Answer from the drawing. Dimensions are ordinates in mm from the lowest x, y and z of the part. A direction names the side the tool comes from. Coordinates: 2 decimals unless noted, no trailing zeros. Write each loop counter-clockwise with the first axis right and the second up, starting at its lowest first coordinate (ties: lowest second). Pieces come first, ordered by that corner, then holes. Notation, with made-up numbers: M -7.75,87.5 L 15.25,87.5 A28 cw 15.25,106.5 Z; hole C 53.5,-26.5 d4. An arc over 180 degrees is marked long. Put each result on its own line as item: value. Start each with the question number.
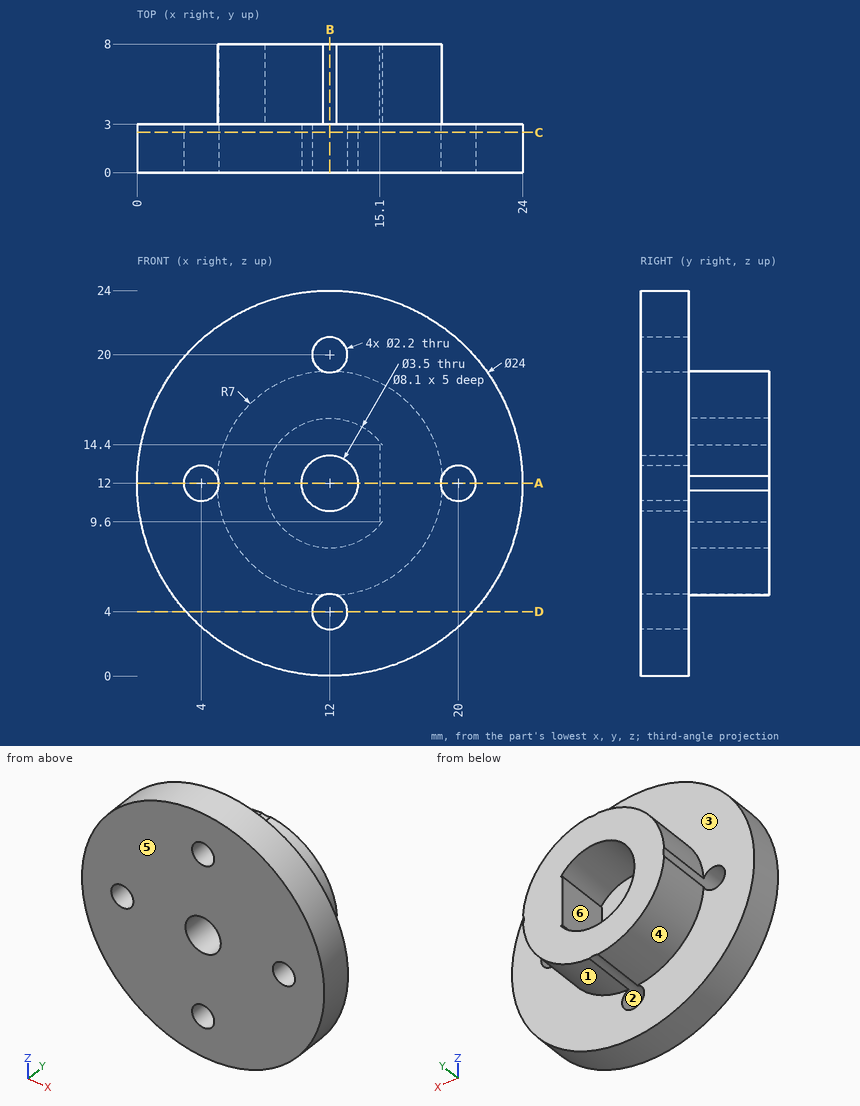
1) Straight lines are drawn through the part: probe 1 along Z at (x, y) = (12, 6); probe 2 along Y at (x, z) = (12.5, 14.5); probe 3 along X at (y, z) = (6.25, 10.25). For each, find the intervals that lie inside material, in ascending order.
2) A cutting plane is placed at A-A on z = 12. Write down the section's boundary in (x, y).
3) A cutting plane is placed at D-D on z = 4. Write down the section's boundary in (x, y).
4) For the marked faces 1, 2 and 3, determine the directions among +Z, -Z, +X, -X, +Y, -Y from which every point of the face is accessible in a straight line to the end or side of a thin tool.
5) Given pin 1 Ø3 at (x, z) = (12, 12) entering from -Y; pin 2 Ø1.5 at (x, y) = (13, 6.5) entering from +Z; pin 3 Ø1 at (y, z) = (1.5, 6) entering from +X; pin 4 Ø2 at (x, z) = (19, 5) entering from +Y, each flat-ended and moving along its own axis, determine where each tip first touches the part or whether it passes through.
6) A cutting plane is placed at C-C on y = 2.5. Write down the section's boundary in (x, z), then the cut area to 3 significant figures.
7) A cutting plane is placed at B-B on x = 12. Write down the section's boundary in (y, z).
8) Determine the mould class of the marked faces 4, 5 and 6 for opening direction X: +X half, -X half, draft (parallel to the pull), parting line (faces both ways), or undercut.
Answers follow:
1. probe 1: z = 5.1 to 7.95, 16.05 to 18.9
1. probe 2: y = 0 to 3
1. probe 3: x = 5.22 to 8.35, 15.1 to 18.78
2. outline: M 0,0 L 2.9,0 L 2.9,3 L 0,3 Z; M 5.1,0 L 10.25,0 L 10.25,3 L 7.95,3 L 7.95,8 L 5.1,8 Z; M 13.75,0 L 18.9,0 L 18.9,8 L 15.1,8 L 15.1,3 L 13.75,3 Z; M 21.1,0 L 24,0 L 24,3 L 21.1,3 Z
3. outline: M 3.06,0 L 10.9,0 L 10.9,3 L 3.06,3 Z; M 13.1,0 L 20.94,0 L 20.94,3 L 13.1,3 Z
4. face 1: -Z, +X, +Y
4. face 2: +Y, -Y
4. face 3: +Y
5. pin 1: passes through
5. pin 2: stops at z = 18.99
5. pin 3: stops at x = 22.67
5. pin 4: stops at y = 3
6. outline: C 12,12 d24; hole C 4,12 d2.2; hole C 12,12 d3.5; hole C 12,4 d2.2; hole C 12,20 d2.2; hole C 20,12 d2.2
6. area: 428 mm²
7. outline: M 0,0 L 3,0 L 3,2.9 L 0,2.9 Z; M 0,5.1 L 8,5.1 L 8,7.95 L 3,7.95 L 3,10.25 L 0,10.25 Z; M 0,13.75 L 3,13.75 L 3,16.05 L 8,16.05 L 8,18.9 L 0,18.9 Z; M 0,21.1 L 3,21.1 L 3,24 L 0,24 Z
8. face 4: -X half
8. face 5: draft
8. face 6: undercut
